Work out the finished part from the listing and answer in its coordinate system (mm). Face numbers are marked on the shaded views. A direction names the side the tool comes from. Give positions to 0.01 mm unless a question says otherwise; leave off trailing zeros. Loops run counter-clockwise (first coordinate to the right, second up) from the corner with the lowest first, then second, coordinate; pieces in that order, holes last.
```python
from build123d import *

# Parameters (mm, degrees)
BOSS_EXTRUDE1_DEPTH = 7.4
CUT_EXTRUDE5_REACH  = 39.59
SKETCH2_W           = 3.6
SKETCH2_H           = 10.3
SKETCH4_R           = 1.725
CUT_EXTRUDE3_DEPTH  = 9
SKETCH3_W           = 5.7
SKETCH3_H           = 2.6
CUT_EXTRUDE4_DEPTH  = 38.589892258
CHAMFER1_SIZE       = 8
FILLET4_R           = 3
FILLET5_R           = 5
FILLET6_R           = 1


with BuildPart() as part:
    # Sketch1 → Boss-Extrude1 (new body)
    with BuildSketch(Plane.XY):
        Polygon((0, 0), (20.2, 0), (20.2, 5.7), (33.2, 5.7), (33.2, 16), (0, 16), align=None)
        with BuildLine():
            Line((25.2, 12.425), (28.2, 12.425))
            ThreePointArc((28.2, 12.425), (29.925, 10.7), (28.2, 8.975))
            Line((28.2, 8.975), (25.2, 8.975))
            ThreePointArc((25.2, 8.975), (23.475, 10.7), (25.2, 12.425))
        make_face(mode=Mode.SUBTRACT)
    extrude(amount=BOSS_EXTRUDE1_DEPTH)

    # Cut-Extrude5: up to this face of the body (flat: up to its plane)
    cut_extrude5_end = Plane(part.part.faces().sort_by_distance((20.2, 2.85, 3.7))[0])
    # Sketch2 → Cut-Extrude5 (cut, up to the picked face)
    with BuildSketch(Plane(origin=(33.2, 0, 0), x_dir=(0, 0, -1), z_dir=(1, 0, 0)), mode=Mode.PRIVATE) as cut_extrude5_sk1:
        with Locations((-1.8, 10.85)):
            Rectangle(SKETCH2_W, SKETCH2_H)
    cut_extrude5_tool1 = split(extrude(cut_extrude5_sk1.sketch, amount=-CUT_EXTRUDE5_REACH, mode=Mode.PRIVATE), bisect_by=cut_extrude5_end, keep=Keep.BOTH, mode=Mode.PRIVATE)
    add(cut_extrude5_tool1.solids().sort_by(Axis((33.2, 10.85, 1.8), (-1, 0, 0)))[0], mode=Mode.SUBTRACT)

    # Sketch4 → Cut-Extrude3 (cut)
    with BuildSketch(Plane.XZ):
        with Locations(Location((15, 4.65, 0), (0, 0, 270))):
            Circle(SKETCH4_R)
        with Locations(Location((5.2, 4.65, 0), (0, 0, 270))):
            Circle(SKETCH4_R)
    extrude(amount=-CUT_EXTRUDE3_DEPTH, mode=Mode.SUBTRACT)

    # Sketch3 → Cut-Extrude4 (cut, through all)
    with BuildSketch(Plane(origin=(0, 0, 0), x_dir=(-1, 0, 0), z_dir=(0, 0, -1))):
        with Locations((-15, 5.3)):
            Rectangle(SKETCH3_W, SKETCH3_H)
        with Locations((-5.2, 5.3)):
            Rectangle(SKETCH3_W, SKETCH3_H)
    extrude(amount=-CUT_EXTRUDE4_DEPTH, mode=Mode.SUBTRACT)

    # Chamfer1
    chamfer1_edges = [part.edges().sort_by_distance(p)[0] for p in [
        (0, 16, 3.7),
    ]]
    chamfer(chamfer1_edges, length=CHAMFER1_SIZE)

    # Fillet4
    fillet4_edges = [part.edges().sort_by_distance(p)[0] for p in [
        (8, 16, 3.7),
        (0, 8, 3.7),
    ]]
    fillet(fillet4_edges, radius=FILLET4_R)

    # Fillet5
    fillet5_edges = [part.edges().sort_by_distance(p)[0] for p in [
        (33.2, 16, 5.5),
        (33.2, 5.7, 5.5),
    ]]
    fillet(fillet5_edges, radius=FILLET5_R)

    # Fillet6
    fillet6_edges = [part.edges().sort_by_distance(p)[0] for p in [
        (20.2, 2.85, 7.4),
        (4, 12, 7.4),
        (0, 3.378679656, 7.4),
        (0.228361402, 7.90540961, 7.4),
        (8.09459039, 15.771638598, 7.4),
        (33.2, 10.85, 7.4),
        (18.721320344, 16, 7.4),
        (31.735533906, 14.535533906, 7.4),
        (31.735533906, 7.164466094, 7.4),
        (24.2, 5.7, 7.4),
    ]]
    fillet(fillet6_edges, radius=FILLET6_R)


solid = part.part
```
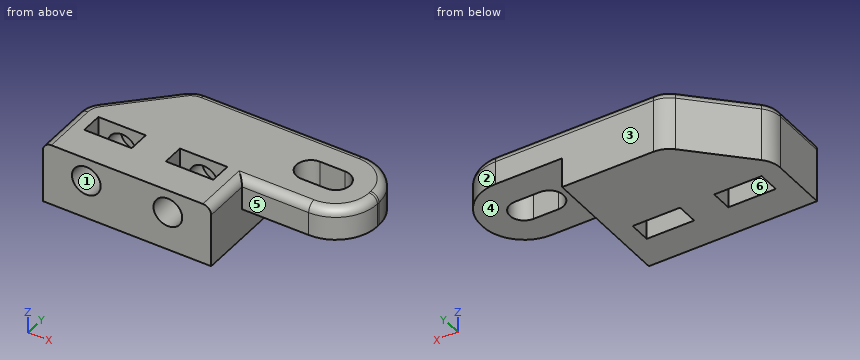
Q1. Which of the six approach directions +Z, -Z, +X, -X, +Y, -Y give full straight-line access (tool end or side, diameter ignored) to the marked faces 4, 5 and 6?
Q2. Section A-A on x = 17.5 is taken. Give the vertices of the cut face in (y, z).
Q3. Section D-D on x = 14 is taken. Give the vertices of the cut face in (y, z).
Q4. Determine the mould class of the marked faces 1, 2 and 3 for opening direction X: +X half, -X half, draft (parallel to the pull), parting line (faces both ways), or undercut.
Q5. Given pin 1 (3.5 mm diameter, centred on x = 27.5, z = 6, fed in from -Y); pin 2 (1.3 mm diameter, centred on y = 5, z = 5.5, fed in from +X); pin 3 (3 mm diameter, centred on x = 26.5, y = 12.5, fed in from -Z); pin 4 (4 mm diameter, centred on x = 15.5, z = 4.5, fed in from -Y), each flat-ended and moving along its own axis, determine where each tip first touches the part or whether it passes through.
Q6. Section C-C on y = 2.75 is taken. Give the vertices of the cut face in (x, z) (3 decimals).
Q7. Section B-B on z = 1.5 is taken. Give the vertices of the cut face in (x, y).
Q8. Consider line 1 along X through (y, z) = (1.7, 4.65) (3 decimals); line 2 along X through (y, z) = (5, 5); line 3 along Y through (x, z) = (12.5, 6.5). Determine where each line is inside the solid, lowest interval first.
Check result:
1. face 4: -Z, +X, +Y, -Y
1. face 5: +Z, -Z, +X, -Y
1. face 6: +Z, -Z
2. outline: (0, 0) - (4, 0) - (4, 7.4) - (0, 7.4) - close; (6.6, 0) - (16, 0) - (16, 6.4) arc R1 ccw to (15, 7.4) - (6.6, 7.4) - close
3. outline: (0, 0) - (4, 0) - (4, 3.24) - (0, 3.24) - close; (0, 6.06) - (4, 6.06) - (4, 7.4) - (0, 7.4) - close; (6.6, 0) - (16, 0) - (16, 6.4) arc R1 ccw to (15, 7.4) - (6.6, 7.4) - (6.6, 6.06) - (9, 6.06) - (9, 3.24) - (6.6, 3.24) - close
4. face 1: undercut
4. face 2: +X half
4. face 3: draft
5. pin 1: stops at y = 5.7
5. pin 2: stops at x = 20.2
5. pin 3: stops at z = 3.6
5. pin 4: stops at y = 0
6. outline: (0, 0) - (20.2, 0) - (20.2, 6.4) arc R1 ccw to (19.2, 7.4) - (1, 7.4) arc R1 ccw to (0, 6.4) - close; hole circle Ø3.45 at (5.2, 4.65); hole circle Ø3.45 at (15, 4.65)
7. outline: (0, 0) - (20.2, 0) - (20.2, 16) - (9.24, 16) arc R3 ccw to (7.12, 15.12) - (0.88, 8.88) arc R3 ccw to (0, 6.76) - close; hole (2.35, 4) - (8.05, 4) - (8.05, 6.6) - (2.35, 6.6) - close; hole (12.15, 4) - (17.85, 4) - (17.85, 6.6) - (12.15, 6.6) - close
8. line 1: x = 0 to 3.475, 6.925 to 13.275, 16.725 to 20.2
8. line 2: x = 0 to 2.35, 8.05 to 12.15, 17.85 to 20.2
8. line 3: y = 0 to 4, 6.6 to 15.99
